Can you work these out from the model? Positions are in its coordinate system, mm. A direction names the side the tool comes from. Give positions to 0.01 mm unless a question says otherwise; leave off trailing zeros. Order: outer loops, then holes, each group sorted by start corner. A loop starts at its lowest first (then second) coordinate and runs counter-clockwise, first axis right, second up.
Item 1: I want a section at C-C, the plane z = 28. Count the separate pieces of the cut face and the enclosed holes in it, then the cut area to 3 significant figures.
Item 2: I want a section at B-B, the plane x = 22. Write out the boundary of the cut face in (y, z), then the cut area to 3 significant figures.
Item 3: I want a section at A-A, the plane y = 0. Write out the boundary of the cut face in (x, z), then the cut area to 3 significant figures.
Item 4: I'm going to push flat-ended pins straight in: pin 1 Ø3 at (x, y) = (35, 30) entering from +Z; pin 2 Ø8 at (x, y) = (35, -10) entering from +Z; pin 3 Ø8 at (x, y) = (12, -5.5) entering from +Z; pin 4 Ø1 at (y, z) = (-16, 22.5) entering from -X. Where does each tip first touch, or does it pass through?
Item 5: If I drill on line 1 along Y through (x, z) = (7, 32.9); line 2 along Y through (x, z) = (7.5, 3.5); line 3 along Y through (x, z) = (0, 27), over which ranges is the centre line in solid material (lowest first)?
Item 6: I want a section at D-D, the plane y = -47.5. Write out the boundary of the cut face in (x, z), then the cut area to 3 significant figures.
Item 7: Which directions (+Z, -Z, +X, -X, +Y, -Y) give clear straight access to the entire face, cutting with the end or side of a thin tool? Please do faces 1 (the flat face through (20, 0, 30.7)), 2 (the cylindrical face through (-47.673, -14.568, 17.086)), 3 (the flat face through (15, 8, 31.95)).
```python
from build123d import *

# Parameters (mm, degrees)
CROQUIS1_R              = 30.25
SALIENTE_EXTRUIR1_DEPTH = 30.7
CROQUIS2_R              = 11
SALIENTE_EXTRUIR2_DEPTH = 3
CROQUIS3_R              = 17.5
CORTAR_EXTRUIR1_DEPTH   = 1.75
CROQUIS4_R              = 2.5
CORTAR_EXTRUIR2_DEPTH   = 87.253637604


with BuildPart() as part:
    # Croquis1 → Saliente-Extruir1 (new body)
    with BuildSketch(Plane.XY):
        with BuildLine():
            Line((0, -52), (60, -52))
            Line((60, -52), (60, 52))
            Line((60, 52), (0, 52))
            ThreePointArc((0, 52), (-52, 0), (0, -52))
        make_face()
        with Locations((7, 0)):
            Circle(CROQUIS1_R, mode=Mode.SUBTRACT)
    extrude(amount=SALIENTE_EXTRUIR1_DEPTH)

    # Croquis2 → Saliente-Extruir2 (add)
    with BuildSketch(Plane.XY.offset(30.7)):
        with BuildLine():
            Line((0, -52), (60, -52))
            Line((60, -52), (60, 52))
            Line((60, 52), (0, 52))
            ThreePointArc((0, 52), (-52, 0), (0, -52))
        make_face()
        with Locations((7, 0)):
            Circle(CROQUIS2_R, mode=Mode.SUBTRACT)
    extrude(amount=SALIENTE_EXTRUIR2_DEPTH)

    # Croquis3 → Cortar-Extruir1 (cut)
    with BuildSketch(Plane.XY.offset(33.7)):
        with Locations((7, 0)):
            Circle(CROQUIS3_R)
    extrude(amount=-CORTAR_EXTRUIR1_DEPTH, mode=Mode.SUBTRACT)

    # Croquis4 → Cortar-Extruir2 (cut, through all)
    with BuildSketch(Plane.XY.offset(33.7)):
        with Locations((35, 30)):
            Circle(CROQUIS4_R)
        with Locations((0, 47.5)):
            Circle(CROQUIS4_R)
        with Locations((-27.919799484, 38.428307233)):
            Circle(CROQUIS4_R)
        with Locations((-45.175184524, 14.678307233)):
            Circle(CROQUIS4_R)
        with Locations((-45.175184524, -14.678307233)):
            Circle(CROQUIS4_R)
        with Locations((-27.919799484, -38.428307233)):
            Circle(CROQUIS4_R)
        with Locations((0, -47.5)):
            Circle(CROQUIS4_R)
        with Locations((35, 10)):
            Circle(CROQUIS4_R)
        with Locations((35, -10)):
            Circle(CROQUIS4_R)
        with Locations((35, -30)):
            Circle(CROQUIS4_R)
    extrude(amount=-CORTAR_EXTRUIR2_DEPTH, mode=Mode.SUBTRACT)


solid = part.part
```
Results list:
1. separate pieces: 1
1. enclosed holes: 9
1. area: 7,440 mm2
2. outline: (-52, 0) - (-26.27, 0) - (-26.27, 30.7) - (26.27, 30.7) - (26.27, 0) - (52, 0) - (52, 33.7) - (9.01, 33.7) - (9.01, 31.95) - (-9.01, 31.95) - (-9.01, 33.7) - (-52, 33.7) - close
2. area: 1,860 mm2
3. outline: (-52, 0) - (-23.25, 0) - (-23.25, 30.7) - (-4, 30.7) - (-4, 31.95) - (-10.5, 31.95) - (-10.5, 33.7) - (-52, 33.7) - close; (18, 30.7) - (37.25, 30.7) - (37.25, 0) - (60, 0) - (60, 33.7) - (24.5, 33.7) - (24.5, 31.95) - (18, 31.95) - close
3. area: 1,830 mm2
4. pin 1: passes through
4. pin 2: stops at z = 33.7
4. pin 3: stops at z = 31.95
4. pin 4: stops at x = -49.64
5. line 1: y = -52 to -17.5, 17.5 to 52
5. line 2: y = -52 to -30.25, 30.25 to 52
5. line 3: y = -52 to -50, -45 to -29.43, 29.43 to 45, 50 to 52
6. outline: (-21.16, 0) - (-2.5, 0) - (-2.5, 33.7) - (-21.16, 33.7) - close; (2.5, 0) - (60, 0) - (60, 33.7) - (2.5, 33.7) - close
6. area: 2,570 mm2
7. face 1: -Z
7. face 2: +Z, -Z
7. face 3: +Z
